Verification items for the finished model (mm, model axes). A direction names the side the tool comes from. Round coordinates to 2 decimals unless told otherwise and drop trailing zeros. Loops run counter-clockwise (first coordinate to the right, second up) from the corner with the lowest first, then second, coordinate; pieces in that order, holes last. Notation, with made-up numbers: M -2.75,58 L 20.25,58 A3 cw 20.25,62 Z; hole C 42.5,-22 d9. An arc over 180 degrees is marked long. One line per item, written item: value.
from build123d import *

# Parameters (mm, degrees)
SKETCH_1_R          = 95
EXTRUDE_1_DEPTH     = 13.208
SKETCH_2_R          = 8.820632657
SKETCH_2_R_2        = 6.280632657
CUT_EXTRUDE_1_DEPTH = 3.302
SKETCH_3_R          = 15.1013679
EXTRUDE_2_DEPTH     = 34.036


with BuildPart() as part:
    # 草图1 → 凸台-拉伸1 (new body)
    with BuildSketch(Plane.XY):
        Circle(SKETCH_1_R)
    extrude(amount=EXTRUDE_1_DEPTH)

    # 草图2 → 切除-拉伸1 (cut)
    with BuildSketch(Plane.XY.offset(13.208)):
        Circle(SKETCH_2_R)
        Circle(SKETCH_2_R_2, mode=Mode.SUBTRACT)
    extrude(amount=-CUT_EXTRUDE_1_DEPTH, mode=Mode.SUBTRACT)

    # 草图3 → 凸台-拉伸2 (add)
    with BuildSketch(Plane.XY.offset(13.208)):
        Circle(SKETCH_3_R)
    extrude(amount=EXTRUDE_2_DEPTH)


solid = part.part
(1) Mould release check, pull along Z, two halves, no side actions. Record for faces 3 (the face through (6, -4, 9.906)), 4 (the face through (-3.274, -14.742, 29.988)), 5 (the face through (0, 0, 47.244)): +Z half, -Z half, draft (parallel to the pull), parting line (faces both ways), or undercut.
Completed:
face 3: undercut
face 4: draft
face 5: +Z half
(2) Sectioned sample at C-C on z = 36. Enter the section's corners in (x, y), and give its area (3 significant figures).
Completed:
outline: C 0,0 d30.2
area: 716 mm^2
(3) Sectioned sample at D-D on x = -26.5. Enter the section's corners in (y, z), and give its area (3 significant figures).
Completed:
outline: M -91.23,0 L 91.23,0 L 91.23,13.21 L -91.23,13.21 Z
area: 2,410 mm^2
(4) Thickness scan on L1, parallel to Y at x = 0, z = 10.75; L2, parallel to Y at x = -5, z = 11; L3, parallel to Z at x = 18.5, y = 18. Record the ranges inside material, lowest first. Write a range as from..to.
Completed:
L1: y = -95..-8.82, -6.28..6.28, 8.82..95
L2: y = -94.87..-7.27, -3.8..3.8, 7.27..94.87
L3: z = 0..13.21
(5) Sectioned sample at A-A on x = 0. Enter the section's corners in (y, z), and give its area (3 significant figures).
Completed:
outline: M -95,0 L 95,0 L 95,13.21 L 15.1,13.21 L 15.1,47.24 L -15.1,47.24 L -15.1,13.21 L -95,13.21 Z; hole M -8.82,9.91 L -6.28,9.91 L -6.28,13.21 L -8.82,13.21 Z; hole M 6.28,9.91 L 8.82,9.91 L 8.82,13.21 L 6.28,13.21 Z
area: 3,520 mm^2
(6) Depth check by flat-ended pin: pin 1 Ø2 at (x, y) = (-21.5, -49) entering from +Z; pin 2 Ø1.5 at (x, z) = (-48.5, 6.5) entering from +Y; pin 3 Ø10 at (x, z) = (-28, 11) entering from -Y. Enter the tip coordinate at first touch or a pass-through.
Completed:
pin 1: stops at z = 13.21
pin 2: stops at y = 82.13
pin 3: stops at y = -92.17
(7) Tool access check on faces 1 (the face through (-1, 1, 0)), 2 (the face through (-1.36, -6.13, 11.58)). Record the directions out of +Z, -Z, +X, -X, +Y, -Y that give a thin tool (end or side, any length) a straight path to the whole face; none if there is none.
Completed:
face 1: -Z, +X, -X, +Y, -Y
face 2: none
